```python
from build123d import *

# Parameters (mm, degrees)
F0_W     = 150
F0_H     = 50.8
F1_DEPTH = 80
F2_W     = 51
F2_H     = 150
F3_DEPTH = 40
F4_R     = 15.425374
F5_DEPTH = 25.4


with BuildPart() as f1:
    # F0 (on Right) → F1 (new body)
    with BuildSketch(Plane.YZ):
        with Locations((15.329447, 25.4)):
            Rectangle(F0_W, F0_H)
    extrude(amount=F1_DEPTH)

    # F2 (on face) → F3 (cut)
    with BuildSketch(Plane.XY.offset(50.8)):
        with Locations((40, 15.329447)):
            Rectangle(F2_W, F2_H)
    extrude(amount=-F3_DEPTH, mode=Mode.SUBTRACT)

    # F4 (on face) → F5 (cut)
    with BuildSketch(Plane.YZ):
        with Locations((-36.535583, 31.488702)):
            Circle(F4_R)
    extrude(amount=F5_DEPTH, mode=Mode.SUBTRACT)


solid = f1.part
```
The listing builds one solid part. Answer for the finished solid, in the listing's coordinates (mm). A direction names the side the tool comes from. Coordinates: 2 decimals unless noted, no trailing zeros. Write each loop counter-clockwise with the first axis right and the second up, starting at its lowest first coordinate (ties: lowest second). Pieces come first, ordered by that corner, then holes. Notation, with made-up numbers: (39.5, 32) -> (95.5, 32) arc R18 ccw to (95.5, 44) -> close; hole circle Ø2 at (87.5, 40). An arc over 180 degrees is marked (long way). Write each question's results on one line, items separated by ' | '. Start each with the question number.
1) A cutting plane is placed at D-D (y = 79). Determine the outline of the cut face in (x, z), then the cut area to 3 significant figures.
2) A tool of negligible diameter and unlimited length cuts with its end or side. For faces 4 (the cylindrical face through (7.15, -21.82, 36.12)), 5 (the flat face through (39, -59.671, 8)), 6 (the flat face through (65.5, 14, 31)), from which of +Z, -Z, +X, -X, +Y, -Y can it reach the whole face along a straight path? Write none if from no direction.
3) Flat-ended cylindrical pins translate along their axes: pin 1 Ø6 at (y, z) = (-33, 32.5) entering from -X; pin 2 Ø12 at (x, y) = (46, -35) entering from +Z. Find the tip coordinate at first contact, or state that the pin passes through.
4) A cutting plane is placed at B-B (y = -42.5). Determine the outline of the cut face in (x, z).
5) For a pull along X with two mould halves and no side action, classify faces 1 (the flat face through (14.5, 14, 31)), 2 (the flat face through (39, 90.329, 8)), 3 (the flat face through (80, 14, 26)) as +X half, -X half, draft (parallel to the pull), parting line (faces both ways), or undercut.
6) Straight lines are drawn through the part: probe 1 along X at (y, z) = (14, 39.5); probe 2 along Z at (x, y) = (55, -5.5); probe 3 along Z at (x, y) = (8, -41). For each, find the intervals that lie inside material, in ascending order.
7) A cutting plane is placed at A-A (z = 13.5). Determine the outline of the cut face in (x, y), then the cut area to 3 significant figures.
8) A cutting plane is placed at C-C (z = 30). Determine the outline of the cut face in (x, y).
Values follow:
1) outline: (0, 0) -> (80, 0) -> (80, 50.8) -> (65.5, 50.8) -> (65.5, 10.8) -> (14.5, 10.8) -> (14.5, 50.8) -> (0, 50.8) -> close | area: 2,020 mm²
2) face 4: -X | face 5: +Z, -Z, +X, -X, -Y | face 6: +Z, +Y, -Y
3) pin 1: x = 65.5 | pin 2: z = 10.8
4) outline: (0, 0) -> (80, 0) -> (80, 50.8) -> (65.5, 50.8) -> (65.5, 10.8) -> (14.5, 10.8) -> (14.5, 17.26) -> (0, 17.26) -> close; (0, 45.71) -> (14.5, 45.71) -> (14.5, 50.8) -> (0, 50.8) -> close
5) face 1: undercut | face 2: draft | face 3: +X half
6) probe 1: 0 to 14.5, 65.5 to 80 | probe 2: 0 to 10.8 | probe 3: 0 to 16.72, 46.25 to 50.8
7) outline: (0, -59.67) -> (14.5, -59.67) -> (14.5, 90.33) -> (0, 90.33) -> close; (65.5, -59.67) -> (80, -59.67) -> (80, 90.33) -> (65.5, 90.33) -> close | area: 4,350 mm²
8) outline: (0, -59.67) -> (14.5, -59.67) -> (14.5, -51.89) -> (0, -51.89) -> close; (0, -21.18) -> (14.5, -21.18) -> (14.5, 90.33) -> (0, 90.33) -> close; (65.5, -59.67) -> (80, -59.67) -> (80, 90.33) -> (65.5, 90.33) -> close
